Here's how the part is built. I have some questions about the finished solid (model axes, mm). Face numbers are marked on the shaded views. Give positions to 0.01 mm unless a question says otherwise; leave off trailing zeros. Loops run counter-clockwise (first coordinate to the right, second up) from the corner with the lowest first, then second, coordinate; pieces in that order, holes last. Notation, with made-up numbers: (46.25, 30) - (93.25, 30) arc R18 ccw to (93.25, 61) - close; hole circle Ø7 at (35, 70.25). An arc over 180 degrees is marked (long way). Use one line per item in the form item = value.
Autodesk Inventor part; units mm, degrees
ref_plane "YZ Plane" through (0, 0, 0) normal (1, 0, 0) x (0, 1, 0)
ref_plane "XZ Plane" through (0, 0, 0) normal (0, 1, 0) x (-1, 0, 0)
ref_plane "XY Plane" through (0, 0, 0) normal (0, 0, 1) x (1, 0, 0)
sketch "Sketch1" plane through (0, 0, 0) normal (0, 1, 0) x (-1, 0, 0)
  line L0 (52.5, 85) -> (-52.5, 85)
  line L1 (-52.5, 85) -> (-52.5, -85)
  line L2 (-52.5, -85) -> (52.5, -85)
  line L3 (52.5, -85) -> (52.5, 85)
  line L4 (52.5, 85) -> (-52.5, -85) construction
  line L5 (-52.5, 85) -> (52.5, -85) construction
  point P0 (0, 0)
  dimension "d0" = 170
  dimension "d1" = 105
extrude "Extrusion1" add sketch "Sketch1" along normal blind 4
sketch "Sketch2" plane through (0, 4, 0) normal (0, 1, 0) x (1, 0, 0)
  line L0 (-44, 79) -> (44, 79)
  line L1 (44, 79) -> (44, -45)
  line L2 (44, -45) -> (-44, -45)
  line L3 (-44, -45) -> (-44, 79)
  line L4 (52.5, 85) -> (-52.5, 85)
  point P0 (0, 0)
  point P1 (0, 79)
  dimension "d4" = 124
  dimension "d5" = 88
  dimension "d6" = 6
extrude "Extrusion2" cut sketch "Sketch2" against normal blind 2
sketch "Sketch3" plane through (0, 4, 0) normal (0, 1, 0) x (1, 0, 0)
  line L0 (-49, -49.5) -> (49, -49.5)
  line L1 (49, -49.5) -> (49, -81.5)
  line L2 (49, -81.5) -> (-49, -81.5)
  line L3 (-49, -81.5) -> (-49, -49.5)
  line L4 (-52.5, 85) -> (-52.5, -85)
  line L5 (-52.5, -85) -> (52.5, -85)
  point P0 (0, 0)
  point P1 (0, -49.5)
  dimension "d9" = 3.5
  dimension "d10" = 3.5
  dimension "d11" = 32
extrude "Extrusion3" add sketch "Sketch3" along normal blind 3
fillet "Fillet1" radius 8 9 edges at (52.5, 2, 85) (-52.5, 2, 85) (52.5, 2, -85) (-52.5, 2, -85) (-44, 3, -79) (44, 3, -79) (-49, 5.5, 49.5) (-49, 5.5, 81.5) (49, 5.5, 81.5)
sketch "Sketch4" plane through (0, 0, 0) normal (0, -1, 0) x (1, 0, 0)
  line L0 (48.5, -79) -> (-48.5, -79) construction
  line L1 (-48.5, -79) -> (-48.5, 43) construction
  line L2 (-48.5, 43) -> (48.5, 43) construction
  line L3 (48.5, 43) -> (48.5, -79) construction
  line L4 (52.5, 77) -> (52.5, -77)
  line L5 (44.5, -85) -> (-44.5, -85) construction
  point P0 (0, 0)
  point P1 (0, -79)
  dimension "d15" = 4
  dimension "d16" = 122
  dimension "d17" = 6
hole "Hole1" at (48.5, 0, -79) at (-48.5, 0, -79) at (-48.5, 0, 43) at (48.5, 0, 43) direction (0, 1, 0) diameter 3.4 depth 8 tip angle 118 countersink diameter 6.3 countersink angle 90
sketch "Sketch5" plane through (0, 2, 0) normal (0, 1, 0) x (1, 0, 0)
  arc A0 (-2, 71) -> (2, 71) centre (0, 67.5359) ccw
  line L0 (-2, 71) -> (-2, 77)
  line L1 (-2, 77) -> (2, 77)
  line L2 (2, 77) -> (2, 71)
  line L3 (-36, 79) -> (36, 79)
  point P0 (0, 0)
  point P1 (0, 77)
  dimension "d25" = 4
  dimension "d26" = 4
  dimension "d27" = 6
  dimension "d28" = 2
extrude "Extrusion4" cut sketch "Sketch5" against normal blind 10
sketch "Sketch6" plane through (0, 7, 0) normal (0, 1, 0) x (1, 0, 0)
  line L0 (-41, -81.5) -> (41, -81.5)
  line L1 (-33.15, -81.5) -> (-26.15, -81.5)
  line L2 (-26.15, -81.5) -> (-26.15, -75)
  line L3 (-26.15, -75) -> (-33.15, -75)
  line L4 (-33.15, -75) -> (-33.15, -81.5)
  line L5 (-49, -57.5) -> (-49, -73.5)
  point P0 (0, 0)
  dimension "d31" = 15.85
  dimension "d32" = 7
  dimension "d33" = 6.5
extrude "Extrusion5" cut sketch "Sketch6" against normal up to surface (3 mm away)
sketch "Sketch7" plane through (0, 7, 0) normal (0, 1, 0) x (1, 0, 0)
  line L0 (-36, -74) -> (36, -74)
  line L1 (36, -74) -> (36, -72)
  line L2 (36, -72) -> (-36, -72)
  line L3 (-36, -72) -> (-36, -74)
  line L4 (-26.15, -81.5) -> (41, -81.5)
  point P0 (0, 0)
  point P1 (0, -72)
  dimension "d36" = 72
  dimension "d37" = 2
  dimension "d38" = 7.5
extrude "Extrusion6" cut sketch "Sketch7" against normal blind 2
properties part number "Top"
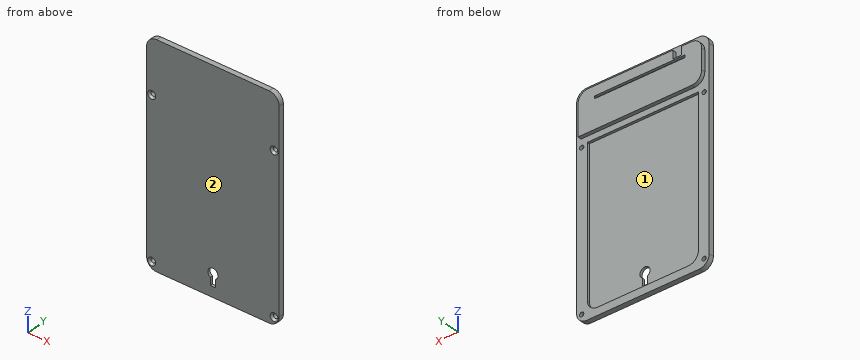
(1) If we section it at B-B (z = 43): List the corners of the cut face in (x, y) for me, plus the area to 3 significant figures.
Geometry says:
outline = (-52.5, 0) - (-51.65, 0) - (-50.2, 1.45) - (-50.2, 4) - (-52.5, 4) - close; (-46.8, 1.45) - (-45.35, 0) - (45.35, 0) - (46.8, 1.45) - (46.8, 4) - (44, 4) - (44, 2) - (-44, 2) - (-44, 4) - (-46.8, 4) - close; (50.2, 1.45) - (51.65, 0) - (52.5, 0) - (52.5, 4) - (50.2, 4) - close
area = 213 mm²
(2) Thinking about a two-plate mould opening in Z: for the marked faces 1 and 2, which applies, pulls with the +Z half, pulls with the -Z half, needs draft (parallel to the pull), parting line crosses it, or undercut?
Geometry says:
face_1 = undercut
face_2 = needs draft
(3) If we section it at C-C (z = -16): List the corners of the cut face in (x, y) for me, plus the area to 3 significant figures.
Geometry says:
outline = (-52.5, 0) - (52.5, 0) - (52.5, 4) - (44, 4) - (44, 2) - (-44, 2) - (-44, 4) - (-52.5, 4) - close
area = 244 mm²
(4) If I drill on probe 1 along X at (y, z) = (3.4, 43); probe 2 along Z at (x, y) = (-21, 2.75); probe 3 along X at (y, z) = (2.25, 6), over which ranges is the centre line in solid material (lowest first)?
Geometry says:
probe_1 = -52.5 to -50.2, -46.8 to -44, 44 to 46.8, 50.2 to 52.5
probe_2 = -85 to -79, 45 to 85
probe_3 = -52.5 to -44, 44 to 52.5
(5) If we section it at A-A (x = 0): List the corners of the cut face in (y, z) for me, plus the area to 3 significant figures.
Geometry says:
outline = (0, -85) - (4, -85) - (4, -79) - (2, -79) - (2, -77) - (0, -77) - close; (0, -63.54) - (2, -63.54) - (2, 45) - (4, 45) - (4, 49.5) - (7, 49.5) - (7, 72) - (5, 72) - (5, 74) - (7, 74) - (7, 81.5) - (4, 81.5) - (4, 85) - (0, 85) - close
area = 497 mm²
(6) For P1, Ø10, axis at x = -6.5, z = -32.5, coming from the -Y side; P2, Ø1, axis at x = 11.5, z = 27.5, coming from the +Y side; P3, Ø0.6, axis at x = 14, y = 6.5, coming from the +Z side; P4, Ø4.5, axis at x = 48.5, z = 43, coming from the -Y side, each with a flat end and sliding along its axis, tell me the tip position at first contact or that it passes through.
Geometry says:
P1 = 0
P2 = 2
P3 = 81.5
P4 = 0.9
